Study the drawing (mm; zero at the part's minimum x, y, z) and answer. A direction names the side the tool comes from. Coordinates: 2 decimals unless noted, no trailing zeros. Write each loop counter-clockwise with the first axis right and the second up, starting at its lowest first coordinate (ties: lowest second). Pieces come first, ordered by that corner, then holes. Notation, with made-up numbers: M 4,35 L 57,35 A19 ccw 57,48 Z; hole C 22,83 d7. An arc over 180 degrees is marked long. Answer as a JSON object with one key per item and string values. Group by question number.
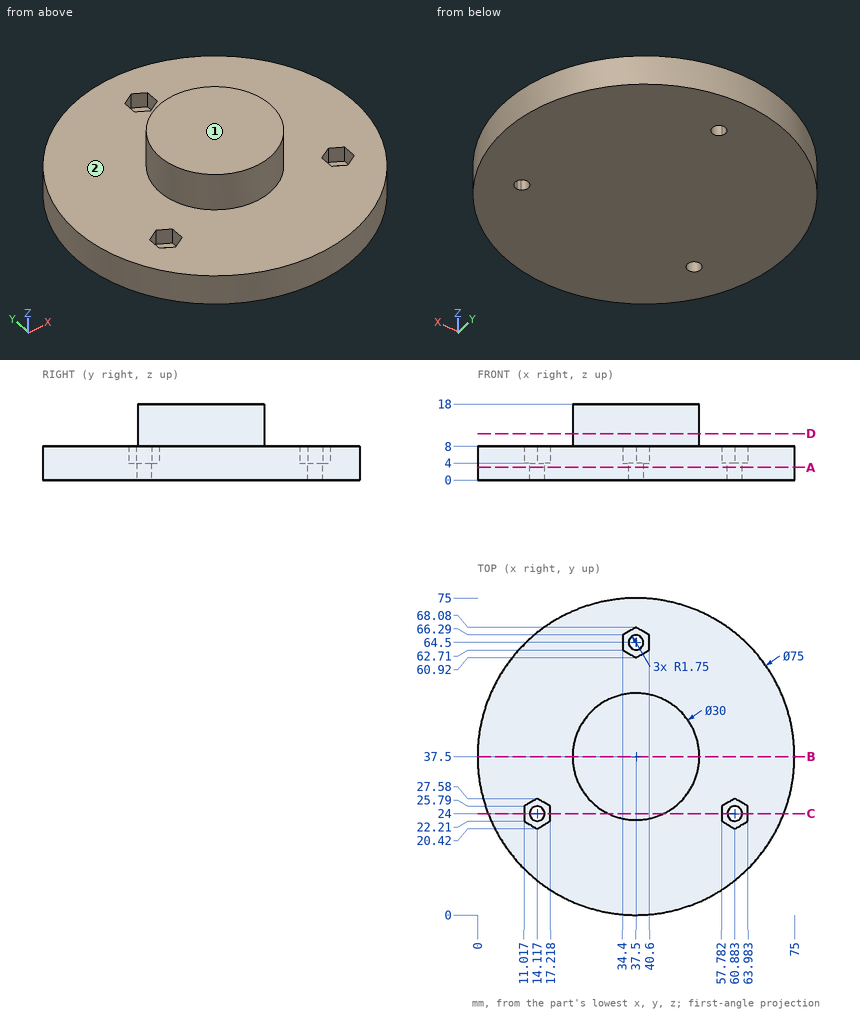
Item 1: A cutting plane is placed at D-D, the plane z = 11. Write down the section's boundary in (x, y).
Item 2: A cutting plane is placed at C-C, the plane y = 24. Write down the section's boundary in (x, z) (1 decimal).
Item 3: A tool of negligible diameter and unlimited length cuts with its end or side. For the marked faces 1 and 2, from which of +Z, -Z, +X, -X, +Y, -Y can it reach the whole face along a straight path? Write none if from no direction.
Item 4: A cutting plane is placed at A-A, the plane z = 3. State how many separate pieces and enclosed holes the cut face has, and give its area (3 significant figures).
Item 5: Flat-ended cylindrical pins translate along their axes: pin 1 Ø4 at (x, y) = (34, 49) entering from -Z; pin 2 Ø1.1 at (y, z) = (23.5, 6) entering from +X (1 decimal); pin 3 Ø7 at (x, y) = (15, 22.5) entering from +Z; pin 4 Ø3 at (y, z) = (64.5, 6.5) entering from +X (1 decimal). Find the tip coordinate at first contact, or state that the pin passes through.
Item 6: Consider L1, parallel to Z at x = 26, y = 59; L2, parallel to X at y = 67, z = 7.25; L3, parallel to Y at x = 61, z = 2.25 (1 decimal). Determine where each line is inside the solid, lowest interval first. Write a range as from..to.
Item 7: A cutting plane is placed at B-B, the plane y = 37.5. Write down the section's boundary in (x, z).
Answer:
{
 "1": {"outline": "C 37.5,37.5 d30"},
 "2": {"outline": "M 2.5,0 L 12.4,0 L 12.4,4 L 11,4 L 11,8 L 2.5,8 Z; M 15.9,0 L 59.1,0 L 59.1,4 L 57.8,4 L 57.8,8 L 44,8 L 44,18 L 31,18 L 31,8 L 17.2,8 L 17.2,4 L 15.9,4 Z; M 62.6,0 L 72.5,0 L 72.5,8 L 64,8 L 64,4 L 62.6,4 Z"},
 "3": {"face 1": "+Z, +X, -X, +Y, -Y", "face 2": "+Z"},
 "4": {"separate pieces": "1", "enclosed holes": "3", "area": "4,390 mm2"},
 "5": {"pin 1": "z = 0", "pin 2": "x = 72.5", "pin 3": "z = 8", "pin 4": "x = 65"},
 "6": {"L1": "0..8", "L2": "14.35..35.63, 39.37..60.65", "L3": "8.3..22.3, 25.7..66.7"},
 "7": {"outline": "M 0,0 L 75,0 L 75,8 L 52.5,8 L 52.5,18 L 22.5,18 L 22.5,8 L 0,8 Z"}
}
